Geometry check sheet. Reference: the model listing, model coordinates, mm. A direction names the side the tool comes from. Give positions to 0.01 mm unless a question says otherwise; leave off trailing zeros. Write item = value, one per line. Start each with the question number.
1. Mould release check, pull along Y, two halves, no side actions. Record for faces 6 (the flat face through (92.101, 21.551, 1.232)), 7 (the flat face through (28.47, 99.16, 1.23)), 8 (the conical face through (38.624, 59.971, 2.656)): pulls with the +Y half, pulls with the -Y half, needs draft (parallel to the pull), parting line crosses it, or undercut.
2. Thickness scan on line 1 along X through (y, z) = (84, 3.7); line 2 along X through (y, z) = (65, 0.45); line 3 along Y through (x, z) = (34, 4.15). Record the ranges inside material, lowest first.
3. Depth check by flat-ended pin: P1, Ø3, axis at x = 65, z = 0.5, coming from the -Y side; P2, Ø1, axis at y = 86.5, z = 2.5, coming from the -X side; P3, Ø1, axis at x = 61, y = 54.5, coming from the +Z side. Enter the tip coordinate at first touch or a pass-through.
4. Set-up check for faces 1 (the flat face through (70, 61, 5)), 2 (the flat face through (89.973, 101.1, 1.232)), 3 (the flat face through (101.03, 30.98, 3.77)), 4 (the flat face through (28.47, 99.16, 3.77)), 5 (the flat face through (92.101, 21.551, 3.768)): record each of +Z, -Z, +X, -X, +Y, -Y from which the full face is reachable in a straight line by a thin tool's end or side.
```python
from build123d import *

# Parameters (mm, degrees)
F0_R     = 5.9800521353
F1_DEPTH = 5
F2_SIZE  = 2.49999


# Not quite as in the source:
# - a fillet or chamfer is up to 0.001 mm smaller than in the source, because OpenCascade refuses the exact size


with BuildPart() as f1:
    # F0 (on Top) → F1 (new body)
    with BuildSketch(Plane.XY):
        with BuildLine():
            Line((27.7623478323, 49.0298643708), (11.5457307547, 9.5314830542))
            Line((11.5457307547, 9.5314830542), (50.2365343273, 27.6623163372))
            ThreePointArc((50.2365343273, 27.6623163372), (60.7722385086, 38.8133091708), (72.0498927169, 28.4132986261))
            Line((72.0498927169, 28.4132986261), (111.7447488987, 12.1160160238))
            Line((111.7447488987, 12.1160160238), (92.3213660153, 51.5245050192))
            ThreePointArc((92.3213660153, 51.5245050192), (81.6154488918, 62.0616839697), (92.3213660153, 72.5988629201))
            Line((92.3213660153, 72.5988629201), (108.314871788, 111.5538179874))
            Line((108.314871788, 111.5538179874), (69.9733346701, 92.6563069494))
            ThreePointArc((69.9733346701, 92.6563069494), (58.8159662766, 82.4438797358), (47.6585978831, 92.6563069494))
            Line((47.6585978831, 92.6563069494), (9.7151305526, 108.2345321774))
            Line((9.7151305526, 108.2345321774), (27.7623478323, 70.4347789288))
            ThreePointArc((27.7623478323, 70.4347789288), (38.47065847, 59.7323216498), (27.7623478323, 49.0298643708))
        make_face()
        with Locations((60, 61.2126085907)):
            Circle(F0_R, mode=Mode.SUBTRACT)
    extrude(amount=F1_DEPTH)

    # F2 (size 2.5 in the source; OpenCascade refuses exactly that, so slightly less here)
    f2_edges = [f1.edges().sort_by_distance(p)[0] for p in [
        (28.686864, 100.44542, 5),
        (18.738739, 89.334656, 5),
        (38.470658, 59.732322, 5),
        (19.654039, 29.280674, 5),
        (30.891133, 18.5969, 5),
        (60.772239, 38.813309, 5),
        (91.897321, 20.264657, 5),
        (102.033057, 31.820261, 5),
        (81.615449, 62.061684, 5),
        (100.318119, 92.07634, 5),
        (89.144103, 102.105062, 5),
        (58.815966, 82.44388, 5),
        (54.019948, 61.212609, 5),
        (28.686864, 100.44542, 0),
        (18.738739, 89.334656, 0),
        (38.470658, 59.732322, 0),
        (19.654039, 29.280674, 0),
        (30.891133, 18.5969, 0),
        (60.772239, 38.813309, 0),
        (91.897321, 20.264657, 0),
        (102.033057, 31.820261, 0),
        (81.615449, 62.061684, 0),
        (100.318119, 92.07634, 0),
        (89.144103, 102.105062, 0),
        (58.815966, 82.44388, 0),
        (54.019948, 61.212609, 0),
    ]]
    chamfer(f2_edges, length=F2_SIZE)


solid = f1.part
```
Answers:
q1.face_6 = pulls with the -Y half
q1.face_7 = pulls with the +Y half
q1.face_8 = undercut
q2.line_1 = 22.62 to 51.02, 66.61 to 95.71
q2.line_2 = 39.38 to 52.92, 67.08 to 79.91
q2.line_3 = 21.88 to 49.07, 70.4 to 96.48
q3.P1 = 38.55
q3.P2 = 19.85
q3.P3 = 3.81
q4.face_1 = +Z, +X, -X, +Y, -Y
q4.face_2 = -Z, +Y
q4.face_3 = +Z, +X
q4.face_4 = +Z, +Y
q4.face_5 = +Z, -Y
